Check sheet for the modelled part. Datum: model origin and axes. Units: mm. A direction names the side the tool comes from. Give positions to 0.01 mm unless a question says otherwise; leave off trailing zeros. Loops run counter-clockwise (first coordinate to the right, second up) from the corner with the lowest first, then second, coordinate; pieces in that order, holes last. Notation, with made-up numbers: (27, -36.5) - (61, -36.5) arc R34 ccw to (61, -2.5) - close; hole circle Ø5 at (77.5, 70). An arc over 180 degrees is marked (long way). Use one line per item in the form item = value.
from build123d import *

# Parameters (mm, degrees)
SKETCH1_W             = 93.5
SKETCH1_H             = 90
BOSS_EXTRUDE1_DEPTH   = 5.4
CUT_EXTRUDE1_REACH    = 66.978
SKETCH2_W             = 83.5
SKETCH2_H             = 78
CHAMFER1_SIZE         = 7
CHAMFER2_SIZE         = 7
CHAMFER3_SIZE         = 7
CHAMFER4_SIZE         = 7
CHAMFER5_SIZE         = 7
CHAMFER6_SIZE         = 7
CHAMFER7_SIZE         = 7
CHAMFER8_SIZE         = 7
CUT_EXTRUDE2_REACH    = 67.081
SKETCH4_W             = 2
SKETCH4_H             = 6.295211976
CUT_EXTRUDE3_DEPTH    = 73.5
SKETCH5_R             = 19.9
BOSS_EXTRUDE2_DEPTH   = 10
F_2_CLEARANCE_HOLE1_D = 2.4
F_2_CLEARANCE_HOLE2_D = 2.4
F_2_CLEARANCE_HOLE3_D = 2.4
F_2_CLEARANCE_HOLE4_D = 2.4
HOLE1_D               = 30
FILLET1_R             = 1
FILLET2_R             = 1


with BuildPart() as part:
    # Sketch1 → Boss-Extrude1 (new body)
    with BuildSketch(Plane(origin=(0, 5.4, 0), x_dir=(1, 0, 0), z_dir=(0, 1, 0))):
        Rectangle(SKETCH1_W, SKETCH1_H)
    extrude(amount=-BOSS_EXTRUDE1_DEPTH)

    # Sketch2 → Cut-Extrude1 (cut, up to next)
    with BuildSketch(Plane.XZ.offset(-2), mode=Mode.PRIVATE) as cut_extrude1_sk1:
        Rectangle(SKETCH2_W, SKETCH2_H)
    cut_extrude1_tool1 = extrude(cut_extrude1_sk1.sketch, amount=-CUT_EXTRUDE1_REACH, mode=Mode.PRIVATE) & part.part
    add(cut_extrude1_tool1.solids().sort_by_distance((0, 2, 0))[0], mode=Mode.SUBTRACT)

    # Chamfer1
    chamfer1_edges = [part.edges().sort_by_distance(p)[0] for p in [
        (41.75, 3.7, -39),
    ]]
    chamfer(chamfer1_edges, length=CHAMFER1_SIZE)

    # Chamfer2
    chamfer2_edges = [part.edges().sort_by_distance(p)[0] for p in [
        (41.75, 3.7, 39),
    ]]
    chamfer(chamfer2_edges, length=CHAMFER2_SIZE)

    # Chamfer3
    chamfer3_edges = [part.edges().sort_by_distance(p)[0] for p in [
        (46.75, 2.7, 45),
    ]]
    chamfer(chamfer3_edges, length=CHAMFER3_SIZE)

    # Chamfer4
    chamfer4_edges = [part.edges().sort_by_distance(p)[0] for p in [
        (46.75, 2.7, -45),
    ]]
    chamfer(chamfer4_edges, length=CHAMFER4_SIZE)

    # Chamfer5
    chamfer5_edges = [part.edges().sort_by_distance(p)[0] for p in [
        (-46.75, 2.7, -45),
    ]]
    chamfer(chamfer5_edges, length=CHAMFER5_SIZE)

    # Chamfer6
    chamfer6_edges = [part.edges().sort_by_distance(p)[0] for p in [
        (-41.75, 3.7, -39),
    ]]
    chamfer(chamfer6_edges, length=CHAMFER6_SIZE)

    # Chamfer7
    chamfer7_edges = [part.edges().sort_by_distance(p)[0] for p in [
        (-46.75, 2.7, 45),
    ]]
    chamfer(chamfer7_edges, length=CHAMFER7_SIZE)

    # Chamfer8
    chamfer8_edges = [part.edges().sort_by_distance(p)[0] for p in [
        (-41.75, 3.7, 39),
    ]]
    chamfer(chamfer8_edges, length=CHAMFER8_SIZE)

    # Sketch3 → Cut-Extrude2 (cut, up to next)
    with BuildSketch(Plane.XZ.offset(-0.4), mode=Mode.PRIVATE) as cut_extrude2_sk1:
        Polygon((-41.75, -32), (-35.045211976, -38.704788024), (35.045211976, -38.704788024), (41.75, -32), (41.75, 32), (34.75, 39), (-34.75, 39), (-41.75, 32), align=None)
    cut_extrude2_tool1 = extrude(cut_extrude2_sk1.sketch, amount=-CUT_EXTRUDE2_REACH, mode=Mode.PRIVATE) & part.part
    add(cut_extrude2_tool1.solids().sort_by_distance((0, 0.4, 0.125192))[0], mode=Mode.SUBTRACT)

    # Sketch4 → Cut-Extrude3 (cut)
    with BuildSketch(Plane(origin=(-36.75, 0, 0), x_dir=(0, -1, 0), z_dir=(-1, 0, 0))):
        with Locations((-1, -41.852394012)):
            Rectangle(SKETCH4_W, SKETCH4_H)
    extrude(amount=-CUT_EXTRUDE3_DEPTH, mode=Mode.SUBTRACT)

    # Sketch5 → Boss-Extrude2 (add)
    with BuildSketch(Plane(origin=(0, 10.4, 0), x_dir=(1, 0, 0), z_dir=(0, 1, 0))):
        with Locations(Location((0, 2.404788024, 0), (0, 0, 90))):
            Circle(SKETCH5_R)
    extrude(amount=-BOSS_EXTRUDE2_DEPTH)

    # #2 Clearance Hole1 (through all)
    with Locations(Plane(origin=(0, 5.4, 0), x_dir=(1, 0, 0), z_dir=(0, 1, 0))):
        with Locations((40.871180413, -39.457859948)):
            Hole(F_2_CLEARANCE_HOLE1_D / 2)

    # #2 Clearance Hole2 (through all)
    with Locations(Plane(origin=(0, 5.4, 0), x_dir=(1, 0, 0), z_dir=(0, 1, 0))):
        with Locations((40.871180413, 39.457859948)):
            Hole(F_2_CLEARANCE_HOLE2_D / 2)

    # #2 Clearance Hole3 (through all)
    with Locations(Plane(origin=(0, 5.4, 0), x_dir=(1, 0, 0), z_dir=(0, 1, 0))):
        with Locations((-40.871180413, 39.457859948)):
            Hole(F_2_CLEARANCE_HOLE3_D / 2)

    # #2 Clearance Hole4 (through all)
    with Locations(Plane(origin=(0, 5.4, 0), x_dir=(1, 0, 0), z_dir=(0, 1, 0))):
        with Locations((-40.871180413, -39.457859948)):
            Hole(F_2_CLEARANCE_HOLE4_D / 2)

    # Hole1 (through all)
    with Locations(Plane(origin=(0, 10.4, 0), x_dir=(1, 0, 0), z_dir=(0, 1, 0))):
        with Locations((0, 2.404788024)):
            Hole(HOLE1_D / 2)

    # Fillet1
    fillet1_edges = [part.edges().sort_by_distance(p)[0] for p in [
        (36.75, 1, -38.704788024),
        (-36.75, 1, -38.704788024),
    ]]
    fillet(fillet1_edges, radius=FILLET1_R)

    # Fillet2
    fillet2_edges = [part.edges().sort_by_distance(p)[0] for p in [
        (0, 10.4, 17.495211976),
        (15, 10.4, -2.404788024),
    ]]
    fillet(fillet2_edges, radius=FILLET2_R)


solid = part.part
Item 1: Gauge pin test, flat ends, axial feed: P1, Ø4, axis at x = 17.5, z = 23, coming from the +Y side; P2, Ø2, axis at x = 40.87, z = -39.46, coming from the -Y side; P3, Ø1.6, axis at y = 0.5, z = -42.5, coming from the +X side; P4, Ø3, axis at x = -40.87, z = -39.46, coming from the +Y side. Record the tip position at first contact, or that the pin passes through.
Answer block:
P1 = 0.4
P2 = through
P3 = 43.05
P4 = 5.4
Item 2: Section check C-C on z = -28.5. Record the boundary of the cut face in (x, y).
Answer block:
outline = (-46.75, 0) - (46.75, 0) - (46.75, 5.4) - (41.75, 5.4) - (41.75, 0.4) - (-41.75, 0.4) - (-41.75, 5.4) - (-46.75, 5.4) - close
Item 3: Mould release check, pull along X, two halves, no side actions. Record for faces 1 (the face through (-1, 2, -42)), 2 (the face through (46.75, 3, 1)), 3 (the face through (-43.2, 2.74, 41.55)), 4 (the face through (36.75, 1, -42)): released by +X, released by -X, zero draft, split by the parting line, or undercut.
Answer block:
face_1 = undercut
face_2 = released by +X
face_3 = released by -X
face_4 = undercut
Item 4: Access from +Z, -Z, +X, -X, +Y, -Y to the whole of each face (thin tool, end or side, straight path). Record for faces 5 (the face through (-8, 10.4, 12)), 6 (the face through (19.427, 4.963, 1.909)).
Answer block:
face_5 = +Z, -Z, +X, -X, +Y
face_6 = +Y
Item 5: Section check B-B on x = 0. Record the boundary of the cut face in (y, z), then the cut area to 3 significant figures.
Answer block:
outline = (0, -38.7) - (0.4, -38.7) - (0.4, -22.3) - (9.4, -22.3) arc R1 ccw to (10.4, -21.3) - (10.4, -18.4) arc R1 ccw to (9.4, -17.4) - (0, -17.4) - close; (0, 12.6) - (9.4, 12.6) arc R1 ccw to (10.4, 13.6) - (10.4, 16.5) arc R1 ccw to (9.4, 17.5) - (0.4, 17.5) - (0.4, 39) - (5.4, 39) - (5.4, 45) - (0, 45) - close; (2, -45) - (5.4, -45) - (5.4, -39) - (2, -39) - close
area = 169 mm2
Item 6: Section check A-A on x = 29. Record the boundary of the cut face in (y, z), then the cut area to 3 significant figures.
Answer block:
outline = (0, -38.7) - (0.4, -38.7) - (0.4, 39) - (5.4, 39) - (5.4, 45) - (0, 45) - close; (2, -45) - (5.4, -45) - (5.4, -39) - (2, -39) - close
area = 83.9 mm2
Item 7: Thickness scan on L1, parallel to Z at x = -16, y = 5.25; L2, parallel to Z at x = 33.5, y = 5.25; L3, parallel to Z at x = -40.5, y = 1. Record the ranges inside material, lowest first.
Answer block:
L1 = -45 to -39, -14.24 to 9.43, 39 to 45
L2 = -45 to -39, 39 to 45
L3 = -44.25 to -40.6, -38.32 to -33.25, 33.25 to 38.32, 40.6 to 44.25
Item 8: Section check D-D on y = 7.75. Record the boundary of the cut face in (x, z).
Answer block:
outline = circle Ø39.8 at (0, -2.4); hole circle Ø30 at (0, -2.4)
